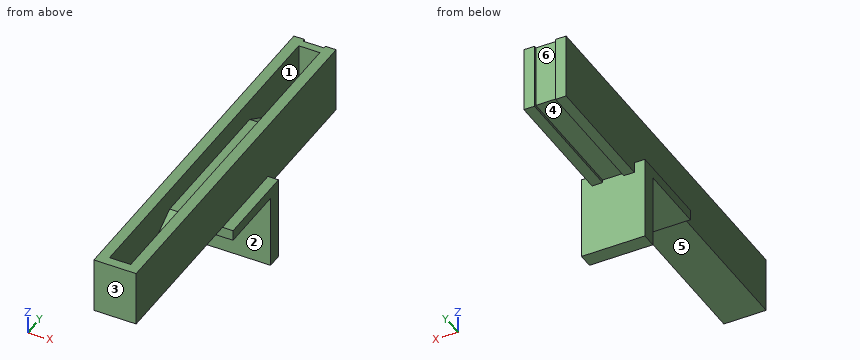
from build123d import *

# Parameters (mm, degrees)
BOSS_EXTRUDE2_DEPTH = 15
BOSS_EXTRUDE3_DEPTH = 5
BOSS_EXTRUDE4_DEPTH = 5
BOSS_EXTRUDE5_DEPTH = 10
SKETCH9_W           = 10
SKETCH9_H           = 4.5
BOSS_EXTRUDE6_DEPTH = 17.8


with BuildPart() as part:
    # Sketch2 → Boss-Extrude2 (new, symmetric)
    with BuildSketch(Plane(origin=(0, 0, 0), x_dir=(0, 0, -1), z_dir=(1, 0, 0))):
        Polygon((0, 0), (0, -40), (5, -40), (5, -7), (40, -7), (40, 0), align=None)
    extrude(amount=BOSS_EXTRUDE2_DEPTH, both=True)

    # Sketch3 → Boss-Extrude3 (add, symmetric)
    with BuildSketch(Plane(origin=(0, 0, 0), x_dir=(0, 0, -1), z_dir=(1, 0, 0))):
        Polygon((0, -116), (-8.5, -116), (-8.5, -71.626882213), (-16.532330081, -58.612316561), (-16.532330081, 11.829172037), (0, 40.464007705), align=None)
    extrude(amount=BOSS_EXTRUDE3_DEPTH, both=True)

    # Sketch4 → Boss-Extrude4 (add)
    with BuildSketch(Plane.ZY.offset(5)):
        Polygon((0, 60), (26.3, 60), (26.3, -116), (0, -116), (0, 0), (-5, 0), (-5, 60), align=None)
    boss_extrude4 = extrude(amount=BOSS_EXTRUDE4_DEPTH)

    # Mirror1: Boss-Extrude4 across plane
    add(boss_extrude4.mirror(Plane(origin=(0, 0, 0), x_dir=(0, 0, 1), z_dir=(1, 0, 0))))

    # Sketch8 → Boss-Extrude5 (add)
    with BuildSketch(Plane.ZY.offset(-5)):
        Polygon((0, 0), (0, 55), (26.3, 55), (26.3, 58.7), (-3.7, 58.7), (-3.7, 0), align=None)
    extrude(amount=BOSS_EXTRUDE5_DEPTH)

    # Sketch9 → Boss-Extrude6 (add)
    with BuildSketch(Plane.XY.offset(8.5)):
        with Locations((0, -113.75)):
            Rectangle(SKETCH9_W, SKETCH9_H)
    extrude(amount=BOSS_EXTRUDE6_DEPTH)


solid = part.part
Design review of the part built by this model. Coordinates are the model's own, in mm. Face numbers are marked on the shaded views. A direction names the side the tool comes from. Coordinates: 2 decimals unless noted, no trailing zeros. Order: outer loops, then holes, each group sorted by start corner. A loop starts at its lowest first (then second) coordinate and runs counter-clockwise, first axis right, second up.
Item 1: Take a section at D-D, the plane y = -94. Write out the cut boundary in (x, z).
Item 2: For line 1 (X direction, y = 7.5, z = 19); line 2 (Y direction, x = 1.25, z = 14.5); line 3 (X direction, y = -66, z = 2), list the stretches that pass through material, from the lowest coordinate up.
Item 3: Take a section at C-C, the plane z = -32.5. Write out the cut boundary in (x, y), then the cut area to 3 significant figures.
Item 4: For the marked faces 1, 2 and 3, list the 3-axis set-ups (+Z, -Z, +X, -X, +Y, -Y) from which the entire face can be reached by the end or side of a thin tool; tool diameter is ignored.
Item 5: Take a section at B-B, the plane x = 3.25. Write out the cut boundary in (y, z), then the cut area to 3 significant figures.
Item 6: The part is to be moulded in two halves that separate along X. For the marked faces 4, 5 and 6, say which applies: pulls with the +X half, pulls with the -X half, needs draft (parallel to the pull), parting line crosses it, or undercut.
Item 7: For pin 1 Ø1.5 at (x, y) = (-13.5, -21) entering from +Z; pin 2 Ø8 at (x, z) = (1.5, -11.5) entering from -Y; pin 3 Ø6 at (y, z) = (-33, 8.5) entering from -X, all flat-tipped, find the tip position at first contact; note any pin that passes through.
Item 8: Take a section at A-A, the plane y = -42. Write out the cut boundary in (x, z), then the cut area to 3 significant figures.
The answers:
1. outline: (-10, 0) - (10, 0) - (10, 26.3) - (5, 26.3) - (5, 8.5) - (-5, 8.5) - (-5, 26.3) - (-10, 26.3) - close
2. line 1: x = -10 to -5, 5 to 10
2. line 2: y = -116 to -111.5, -61.91 to 15.35, 55 to 58.7
2. line 3: x = -10 to 10
3. outline: (-15, -7) - (15, -7) - (15, 0) - (-15, 0) - close
3. area: 210 mm2
4. face 1: +Z
4. face 2: -Z, +X, -X, -Y
4. face 3: +Z, -Z, +X, -X, -Y
5. outline: (-116, 0) - (-40, 0) - (-40, -5) - (-7, -5) - (-7, -40) - (0, -40) - (0, -3.7) - (58.7, -3.7) - (58.7, 26.3) - (55, 26.3) - (55, 0) - (40.46, 0) - (11.83, 16.53) - (-58.61, 16.53) - (-71.63, 8.5) - (-111.5, 8.5) - (-111.5, 26.3) - (-116, 26.3) - close
5. area: 2,780 mm2
6. face 4: undercut
6. face 5: needs draft
6. face 6: undercut
7. pin 1: stops at z = 0
7. pin 2: stops at y = -7
7. pin 3: stops at x = -10
8. outline: (-10, 0) - (10, 0) - (10, 26.3) - (5, 26.3) - (5, 16.53) - (-5, 16.53) - (-5, 26.3) - (-10, 26.3) - close
8. area: 428 mm2
